Design review of the part shown in the three views and the two pictorial views. Dimensions are in mm from the part's minimum x, y and z. Coordinates: 2 decimals unless noted, no trailing zeros. Write each loop counter-clockwise with the first axis right and the second up, starting at its lowest first coordinate (ties: lowest second). Pieces come first, ordered by that corner, then holes. Notation, with made-up numbers: M 0.25,70 L 33.25,70 A19 ccw 33.25,97 Z; hole C 24,12.5 d4. An arc over 180 degrees is marked long. One line per question, with ' | ' between items.
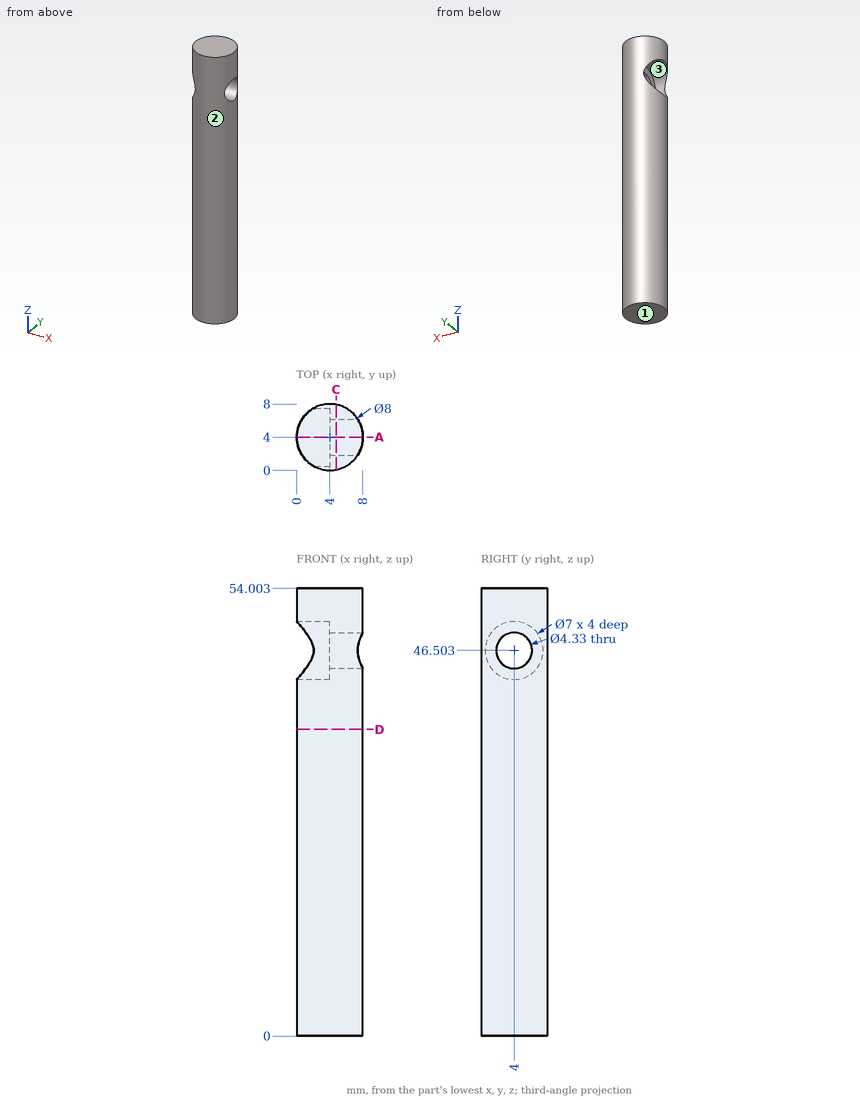
1. For line 1 along Y through (x, z) = (4.25, 22); line 2 along Y through (x, z) = (3.25, 49); line 3 along Z through (x, y) = (5.5, 4.75), list the stretches that pass through material, from the lowest coordinate up.
Computed values:
line 1: y = 0.01 to 7.99 | line 2: y = 0.07 to 1.55, 6.45 to 7.93 | line 3: z = 0 to 44.47, 48.53 to 54
2. Take a section at D-D on z = 37. State the section outline as (x, y) points.
Computed values:
outline: C 4,4 d8
3. Draft analysis for pull direction Y (two halves, no side actions). For the marked faces 1, 2 and 3, state which applies: pulls with the +Y half, pulls with the -Y half, needs draft (parallel to the pull), parting line crosses it, or undercut.
Computed values:
face 1: needs draft | face 2: parting line crosses it | face 3: undercut
4. Take a section at A-A on y = 4. State the section outline as (x, z) points, plus the area to 3 significant figures.
Computed values:
outline: M 0,0 L 8,0 L 8,44.34 L 4,44.34 L 4,43 L 0,43 Z; M 0,50 L 4,50 L 4,48.67 L 8,48.67 L 8,54 L 0,54 Z | area: 387 mm2
5. Clearance check with flat-ended pins moving along their axes: P1, Ø2, axis at y = 5.5, z = 25.5, coming from the +X side; P2, Ø4, axis at y = 4, z = 46.5, coming from the -X side. State where each tip first meets the part, or that it passes through.
Computed values:
P1: stops at x = 7.97 | P2: passes through
6. Take a section at C-C on x = 4.75. State the section outline as (y, z) points (1 decimal).
Computed values:
outline: M 0.1,0 L 7.9,0 L 7.9,54 L 0.1,54 Z; hole C 4,46.5 d4.3
